For this review, take the finished solid that the model builds, in its own axes (mm). Give positions to 0.01 mm unless a question says otherwise; leave off trailing zeros. Write each loop counter-clockwise with the first axis right and the second up, starting at its lowest first coordinate (ties: lowest second). Pieces come first, ordered by that corner, then holes. Notation, with made-up numbers: (40, 42) -> (60, 42) arc R6 cw to (60, 47) -> close; hole circle Ø6 at (19.5, 29). An arc over 180 degrees is marked (long way). Answer as CSV lines item,"result".
```python
from build123d import *

# Parameters (mm, degrees)
F0_R     = 4.5
F1_DEPTH = 10
F2_R     = 2


with BuildPart() as f1:
    # F0 (on Front) → F1 (new body)
    with BuildSketch(Plane.XZ):
        Polygon((14.562795, -11.751718), (17.458684, 6.735892), (2.895889, 18.48761), (-14.562795, 11.751718), (-17.458684, -6.735892), (-2.895889, -18.48761), align=None)
        Circle(F0_R, mode=Mode.SUBTRACT)
    extrude(amount=F1_DEPTH)

    # F2
    f2_edges = [f1.edges().sort_by_distance(p)[0] for p in [
        (2.895889, -5, 18.48761),
        (17.458684, -5, 6.735892),
        (14.562795, -5, -11.751718),
        (-2.895889, -5, -18.48761),
        (-17.458684, -5, -6.735892),
        (-14.562795, -5, 11.751718),
    ]]
    fillet(f2_edges, radius=F2_R)


solid = f1.part
```
Q1. Clearance check with flat-ended pins moving along their axes: pin 1 (10 mm diameter, centred on x = 14, z = 7, fed in from +Y); pin 2 (1.5 mm diameter, centred on x = 3, y = -6, fed in from -Z); pin 3 (1 mm diameter, centred on y = -4.5, z = -11, fed in from -X); pin 4 (3 mm diameter, centred on y = -4.5, z = -13, fed in from -X) (3 decimals). State where each tip first meets the part, or that it passes through.
Answer block:
pin 1,"stops at y = 0"
pin 2,"stops at z = -16.5"
pin 3,"stops at x = -12.79"
pin 4,"stops at x = -11.555"
Q2. To check wall thickness, follow probe 1 along X at (y, z) = (-4, -4); probe 2 along Z at (x, y) = (0.5, -2.25); probe 3 along Z at (x, y) = (1, -7). State the ranges of each line that lie inside material, in increasing order. Write a range as [from, to].
Answer block:
probe 1,"x = [-17.03, -2.06], [2.06, 15.78]"
probe 2,"z = [-17.18, -4.47], [4.47, 17.56]"
probe 3,"z = [-16.98, -4.39], [4.39, 17.76]"
Q3. Add section D-D (z = 6.5). Write out the cut boundary in (x, y).
Answer block:
outline,"(-15.39, -10) -> (17.21, -10) -> (17.21, 0) -> (-15.39, 0) -> close"
Q4. Add section B-B (y = -5.5). Write out the cut boundary in (x, z).
Answer block:
outline,"(-17.28, -5.6) arc R2 ccw to (-16.56, -7.46) -> (-3.79, -17.76) arc R2 ccw to (-1.82, -18.07) -> (13.49, -12.17) arc R2 ccw to (14.74, -10.61) -> (17.28, 5.6) arc R2 ccw to (16.56, 7.46) -> (3.79, 17.76) arc R2 ccw to (1.82, 18.07) -> (-13.49, 12.17) arc R2 ccw to (-14.74, 10.61) -> close; hole circle Ø9 at (0, 0)"
Q5. Add section C-C (x = -3). Write out the cut boundary in (y, z).
Answer block:
outline,"(-10, -18.15) -> (0, -18.15) -> (0, -3.35) -> (-10, -3.35) -> close; (-10, 3.35) -> (0, 3.35) -> (0, 16.21) -> (-10, 16.21) -> close"
Q6. Draft analysis for pull direction Z (two halves, no side actions). For faces 1 (the cylindrical face through (-2.834, -5.07, -18.184)), 2 (the flat face through (-15.993, -4.93, 2.621)), 3 (the cylindrical face through (-0.59, -4.93, 4.46)), state which applies: released by +Z, released by -Z, zero draft, split by the parting line, or undercut.
Answer block:
face 1,"released by -Z"
face 2,"released by +Z"
face 3,"undercut"
Q7. Add section A-A (z = 0). Write out the cut boundary in (x, y), plus the area to 3 significant figures.
Answer block:
outline,"(-16.4, -10) -> (-4.5, -10) -> (-4.5, 0) -> (-16.4, 0) -> close; (4.5, -10) -> (16.4, -10) -> (16.4, 0) -> (4.5, 0) -> close"
area,"238 mm2"
